from build123d import *

# Parameters (mm, degrees)
ESQUISSE1_W             = 17
ESQUISSE1_H             = 59
BOSS_EXTRU_1_DEPTH      = 2
ESQUISSE2_W             = 8.5
ESQUISSE2_H             = 50
BOSS_EXTRU_2_DEPTH      = 6
ESQUISSE4_R             = 2.25
ENL_V_MAT_EXTRU_6_DEPTH = 27
ESQUISSE3_W             = 1.5
ESQUISSE3_H             = 7
ENL_V_MAT_EXTRU_7_DEPTH = 7
ESQUISSE5_R             = 3.75
ENL_V_MAT_EXTRU_8_DEPTH = 6


with BuildPart() as part:
    # Esquisse1 → Boss.-Extru.1 (new body)
    with BuildSketch(Plane.XY):
        with Locations((8.5, -29.5)):
            Rectangle(ESQUISSE1_W, ESQUISSE1_H)
    extrude(amount=BOSS_EXTRU_1_DEPTH)

    # Esquisse2 → Boss.-Extru.2 (add)
    with BuildSketch(Plane.XY.offset(2)):
        with Locations((4.25, -29.5)):
            Rectangle(ESQUISSE2_W, ESQUISSE2_H)
    extrude(amount=BOSS_EXTRU_2_DEPTH)

    # Esquisse4 → Enlèv. mat.-Extru.6 (cut)
    with BuildSketch(Plane.XY.offset(8)):
        with Locations((8.5, -54.5)):
            Circle(ESQUISSE4_R)
        with Locations((8.5, -29.5)):
            Circle(ESQUISSE4_R)
        with Locations((8.5, -4.5)):
            Circle(ESQUISSE4_R)
    extrude(amount=-ENL_V_MAT_EXTRU_6_DEPTH, mode=Mode.SUBTRACT)

    # Esquisse3 → Enlèv. mat.-Extru.7 (cut)
    with BuildSketch(Plane.XY.offset(8)):
        with Locations((2.25, -58)):
            Rectangle(ESQUISSE3_W, ESQUISSE3_H)
        with Locations((3.75, -58)):
            Rectangle(ESQUISSE3_W, ESQUISSE3_H)
        Polygon((4.5, -48), (3, -49.5), (3, -54.5), (4.5, -54.5), (4.5, -50), align=None)
        Polygon((3, -49.5), (3, -42), (3, -41.5), (1.5, -41.5), (1.5, -54.5), (3, -54.5), align=None)
        Polygon((5.5, -41.5), (5.5, -42), (5.5, -47), (4.5, -48), (4.5, -50), (7, -47.5), (7, -41.5), align=None)
        with BuildLine():
            Line((4.25, -38.75), (4.25, -40.75))
            ThreePointArc((4.25, -40.75), (4.934653197, -40.954174967), (5.395643924, -41.5))
            Line((5.395643924, -41.5), (5.5, -41.5))
            Line((5.5, -41.5), (7, -41.5))
            ThreePointArc((7, -41.5), (6.194543648, -39.555456352), (4.25, -38.75))
        make_face()
        with BuildLine():
            Line((1.5, -41.5), (3, -41.5))
            Line((3, -41.5), (3.104356076, -41.5))
            ThreePointArc((3.104356076, -41.5), (3.565346803, -40.954174967), (4.25, -40.75))
            Line((4.25, -40.75), (4.25, -38.75))
            ThreePointArc((4.25, -38.75), (2.305456352, -39.555456352), (1.5, -41.5))
        make_face()
        with BuildLine():
            Line((3, -41.5), (3, -42))
            ThreePointArc((3, -42), (3.026367109, -41.744612945), (3.104356076, -41.5))
            Line((3.104356076, -41.5), (3, -41.5))
        make_face()
        with BuildLine():
            ThreePointArc((5.395643924, -41.5), (5.473632891, -41.744612945), (5.5, -42))
            Line((5.5, -42), (5.5, -41.5))
            Line((5.5, -41.5), (5.395643924, -41.5))
        make_face()
    enl_v_mat_extru_7 = extrude(amount=-ENL_V_MAT_EXTRU_7_DEPTH, mode=Mode.SUBTRACT)

    # Symétrie1: Enlèv. mat.-Extru.7 across plane
    add(enl_v_mat_extru_7.mirror(Plane.ZX.offset(-29.5)), mode=Mode.SUBTRACT)

    # Esquisse5 → Enlèv. mat.-Extru.8 (cut)
    with BuildSketch(Plane.XY.offset(8)):
        with Locations((8.5, -29.5)):
            Circle(ESQUISSE5_R)
        with Locations((8.5, -4.5)):
            Circle(ESQUISSE5_R)
        with Locations((8.5, -54.5)):
            Circle(ESQUISSE5_R)
    extrude(amount=-ENL_V_MAT_EXTRU_8_DEPTH, mode=Mode.SUBTRACT)


solid = part.part
Design review of the part built by this model. Coordinates are the model's own, in mm. A direction names the side the tool comes from. Coordinates: 2 decimals unless noted, no trailing zeros. Write each loop counter-clockwise with the first axis right and the second up, starting at its lowest first coordinate (ties: lowest second). Pieces come first, ordered by that corner, then holes. Notation, with made-up numbers: (60.5, 24.25) - (108.5, 24.25) arc R24 cw to (108.5, 34.25) - close; hole circle Ø5 at (50, 41.5). An arc over 180 degrees is marked (long way). Use one line per item in the form item = value.
Q1. Machinability: for faces 4 (the flat face through (4.5, -53, 5)), 5 (the flat face through (7, -45, 5)), 6 (the cylindrical face through (4.75, -29.42, 5.04)), which of the approach directions +Z, -Z, +X, -X, +Y, -Y give a long, thin tool a straight path to every point of the face, cutting with its end or side? Answer none if there is none.
Taken from the geometry:
face_4 = +Z, -Y
face_5 = +Z
face_6 = +Z, +X
Q2. For probe 1 along X at (y, z) = (-4.5, 1.45); probe 2 along Y at (x, z) = (8.5, 0.75); probe 3 along X at (y, z) = (-44.5, 4), list the stretches that pass through material, from the lowest coordinate up.
Taken from the geometry:
probe_1 = 0 to 1.5, 4.5 to 6.25, 10.75 to 17
probe_2 = -59 to -56.75, -52.25 to -31.75, -27.25 to -6.75, -2.25 to 0
probe_3 = 0 to 1.5, 3 to 5.5, 7 to 8.5
Q3. The part is to be moulded in two halves that separate along X. For faces 1 (the flat face through (4, -29, 8)), 2 (the flat face through (8.5, -17, 5)), 3 (the flat face through (7, -14, 5)), say which applies: +X half, -X half, draft (parallel to the pull), parting line (faces both ways), or undercut.
Taken from the geometry:
face_1 = draft
face_2 = +X half
face_3 = undercut
Q4. Consider section B-B (y = -29.5). Write out the cut boundary in (x, z).
Taken from the geometry:
outline = (0, 0) - (6.25, 0) - (6.25, 2) - (4.75, 2) - (4.75, 8) - (0, 8) - close; (10.75, 0) - (17, 0) - (17, 2) - (10.75, 2) - close
Q5. Consider section A-A (z = 1.5). Write out the cut boundary in (x, y), plus the area to 3 significant figures.
Taken from the geometry:
outline = (0, -59) - (1.5, -59) - (1.5, -41.5) arc R2.75 cw to (7, -41.5) - (7, -47.5) - (4.5, -50) - (4.5, -59) - (17, -59) - (17, 0) - (4.5, 0) - (4.5, -9) - (7, -11.5) - (7, -17.5) arc R2.75 cw to (1.5, -17.5) - (1.5, 0) - (0, 0) - close; (3, -49.5) - (5.5, -47) - (5.5, -42) arc R1.25 ccw to (3, -42) - close; (3, -17) arc R1.25 ccw to (5.5, -17) - (5.5, -12) - (3, -9.5) - close; hole circle Ø4.5 at (8.5, -54.5); hole circle Ø4.5 at (8.5, -29.5); hole circle Ø4.5 at (8.5, -4.5)
area = 826 mm^2
Q6. Consider section D-D (y = -35.5). Write out the cut boundary in (x, z).
Taken from the geometry:
outline = (0, 0) - (17, 0) - (17, 2) - (8.5, 2) - (8.5, 8) - (0, 8) - close
Q7. Consider section C-C (x = 9.25). Write out the cut boundary in (y, z), plus the area to 3 significant figures.
Taken from the geometry:
outline = (-59, 0) - (-56.62, 0) - (-56.62, 2) - (-59, 2) - close; (-52.38, 0) - (-31.62, 0) - (-31.62, 2) - (-52.38, 2) - close; (-27.38, 0) - (-6.62, 0) - (-6.62, 2) - (-27.38, 2) - close; (-2.38, 0) - (0, 0) - (0, 2) - (-2.38, 2) - close
area = 92.5 mm^2
Q8. Insertion check: pin 1 Ø10 at (x, y) = (11.5, -51.5) entering from +Z; pin 2 Ø6 at (x, y) = (12.5, -26.5) entering from +Z; pin 3 Ø4 at (y, z) = (-14.5, 5.5) entering from +X; pin 4 Ø2.5 at (x, y) = (8.5, -29.5) entering from -Z. Each pin has a flat end and moves straight along its axis. Give the tip position at first contact, or say it passes through.
Taken from the geometry:
pin_1 = 8
pin_2 = 2
pin_3 = 8.5
pin_4 = through
